Part model, mm, in its own coordinate system. Round coordinates to 2 decimals unless told otherwise and drop trailing zeros. Order: outer loops, then holes, each group sorted by start corner. A loop starts at its lowest first (then second) coordinate and runs counter-clockwise, first axis right, second up. Notation, with made-up numbers: (65.25, -35) -> (107.25, -35) arc R18 ccw to (107.25, -7) -> close; hole circle Ø9 at (18, 75). An arc over 180 degrees is marked (long way). Answer as a JSON object with one key per item and string values. Group by question number.
```python
from build123d import *

# Parameters (mm, degrees)
SKETCH1_R                                         = 17.9
SKETCH1_R_2                                       = 6.5
BOSS_EXTRUDE1_DEPTH                               = 4.5
CSK_FOR_M2_5_FLAT_HEAD_MACHINE_SCREW2_D           = 2.9
CSK_FOR_M2_5_FLAT_HEAD_MACHINE_SCREW2_DEPTH       = 4.5
CSK_FOR_M2_5_FLAT_HEAD_MACHINE_SCREW2_CSINK_D     = 5.5
CSK_FOR_M2_5_FLAT_HEAD_MACHINE_SCREW2_CSINK_ANGLE = 90
CSK_FOR_M2_5_FLAT_HEAD_MACHINE_SCREW2_TIP         = 0.871247898


with BuildPart() as part:
    # Sketch1 → Boss-Extrude1 (new body)
    with BuildSketch(Plane.XY):
        Circle(SKETCH1_R)
        Circle(SKETCH1_R_2, mode=Mode.SUBTRACT)
    extrude(amount=BOSS_EXTRUDE1_DEPTH)

    # CSK for M2.5 Flat Head Machine Screw2
    with Locations(Plane.XY.offset(4.5)):
        with Locations((-12.5, 0), (12.5, 0)):
            CounterSinkHole(CSK_FOR_M2_5_FLAT_HEAD_MACHINE_SCREW2_D / 2, CSK_FOR_M2_5_FLAT_HEAD_MACHINE_SCREW2_CSINK_D / 2, depth=CSK_FOR_M2_5_FLAT_HEAD_MACHINE_SCREW2_DEPTH, counter_sink_angle=CSK_FOR_M2_5_FLAT_HEAD_MACHINE_SCREW2_CSINK_ANGLE)
            with Locations((0, 0, -(CSK_FOR_M2_5_FLAT_HEAD_MACHINE_SCREW2_DEPTH + CSK_FOR_M2_5_FLAT_HEAD_MACHINE_SCREW2_TIP / 2))):  # 118° drill point
                Cone(0, CSK_FOR_M2_5_FLAT_HEAD_MACHINE_SCREW2_D / 2, CSK_FOR_M2_5_FLAT_HEAD_MACHINE_SCREW2_TIP, mode=Mode.SUBTRACT)


solid = part.part
```
Q1. Drop flat-ended pins along their axis: pin 1 Ø1 at (x, z) = (9.5, 4) entering from -Y; pin 2 Ø3 at (x, y) = (-13.5, -13) entering from -Z; pin 3 Ø4 at (x, y) = (12.5, 0) entering from +Z; pin 4 Ø1 at (x, z) = (10, 2.5) entering from -Y. Give the stop position or say it passes through.
Q2. Band-saw the part on B-B (x = 0). List the corners of the cut face in (y, z).
Q3. Band-saw the part on C-C (z = 1.5). List the corners of the cut face in (x, y), plus the area to 3 significant figures.
Q4. Two-plate mould, pull along X, no slides. Class faces 1 (the cylindrical face through (-5.158, -3.955, 2.218)), 2 (the cylindrical face through (-14.2, -10.9, 2.2)), 3 (the flat face through (8, 0, 0)): +X half, -X half, draft (parallel to the pull), parting line (faces both ways), or undercut.
Q5. Wall check: line 1 (Y direction, x = 0, z = 1.8); line 2 (X direction, y = 1, z = 3.35); line 3 (Y direction, x = -12.5, z = 0.8). Give the ranges that are in metal, low to high. Write a range as [from, to].
Q6. Band-saw the part on D-D (x = -4). List the corners of the cut face in (y, z), plus the area to 3 significant figures.
Q7. Band-saw the part on A-A (y = 0). List the corners of the cut face in (x, z).
Completed:
{
 "1": {"pin 1": "y = -15.47", "pin 2": "z = 0", "pin 3": "z = 3.75", "pin 4": "y = -15.17"},
 "2": {"outline": "(-17.9, 0) -> (-6.5, 0) -> (-6.5, 4.5) -> (-17.9, 4.5) -> close; (6.5, 0) -> (17.9, 0) -> (17.9, 4.5) -> (6.5, 4.5) -> close"},
 "3": {"outline": "circle Ø35.8 at (0, 0); hole circle Ø2.9 at (-12.5, 0); hole circle Ø13 at (0, 0); hole circle Ø2.9 at (12.5, 0)", "area": "861 mm2"},
 "4": {"face 1": "undercut", "face 2": "parting line", "face 3": "draft"},
 "5": {"line 1": "[-17.9, -6.5], [6.5, 17.9]", "line 2": "[-17.87, -13.75], [-11.25, -6.42], [6.42, 11.25], [13.75, 17.87]", "line 3": "[-12.81, -1.45], [1.45, 12.81]"},
 "6": {"outline": "(-17.45, 0) -> (-5.12, 0) -> (-5.12, 4.5) -> (-17.45, 4.5) -> close; (5.12, 0) -> (17.45, 0) -> (17.45, 4.5) -> (5.12, 4.5) -> close", "area": "111 mm2"},
 "7": {"outline": "(-17.9, 0) -> (-13.95, 0) -> (-13.95, 3.2) -> (-15.25, 4.5) -> (-17.9, 4.5) -> close; (-11.05, 0) -> (-6.5, 0) -> (-6.5, 4.5) -> (-9.75, 4.5) -> (-11.05, 3.2) -> close; (6.5, 0) -> (11.05, 0) -> (11.05, 3.2) -> (9.75, 4.5) -> (6.5, 4.5) -> close; (13.95, 0) -> (17.9, 0) -> (17.9, 4.5) -> (15.25, 4.5) -> (13.95, 3.2) -> close"}
}
